The listing builds one solid part. Answer for the finished solid, in the listing's coordinates (mm). Face numbers are marked on the shaded views. A direction names the side the tool comes from. Coordinates: 2 decimals unless noted, no trailing zeros. Loops run counter-clockwise (first coordinate to the right, second up) from the corner with the lowest first, then second, coordinate; pieces in that order, holes last. Notation, with made-up numbers: M -29,-10.75 L -12,-10.75 A18 cw -12,0.25 Z; hole C -17.5,55.5 d5. An arc over 180 degrees is marked long. Answer in a Markdown table with one row per item. Add a question column.
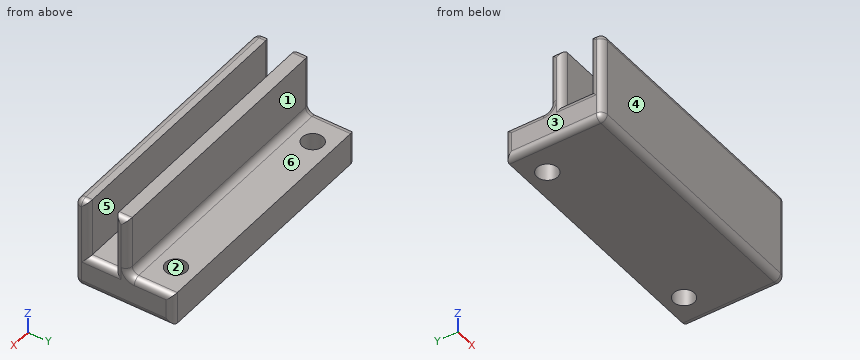
from build123d import *

# Parameters (mm, degrees)
SKETCH2_W           = 40
SKETCH2_H           = 6.9
SKETCH2_R           = 1.6
SKETCH2_H_2         = 2
SKETCH2_H_3         = 4.1
BOSS_EXTRUDE1_DEPTH = 5
SKETCH2_3_W         = 40
SKETCH2_3_H         = 2
BOSS_EXTRUDE2_DEPTH = 14
FILLET1_R           = 1


with BuildPart() as part:
    # Sketch2 → Boss-Extrude1 (new body)
    # profile 1 of 4: a face of its own
    with BuildSketch(Plane.XY):
        with Locations((0, 4.05)):
            Rectangle(SKETCH2_W, SKETCH2_H)
        with Locations((-15, 4.5)):
            Circle(SKETCH2_R, mode=Mode.SUBTRACT)
        with Locations((15, 4.5)):
            Circle(SKETCH2_R, mode=Mode.SUBTRACT)
    # profile 2 of 4: a face of its own
    with BuildSketch(Plane.XY):
        with Locations((0, -0.4)):
            Rectangle(SKETCH2_W, SKETCH2_H_2)
    # profile 3 of 4: a face of its own
    with BuildSketch(Plane.XY):
        with Locations((0, -3.45)):
            Rectangle(SKETCH2_W, SKETCH2_H_3)
    # profile 4 of 4: a face of its own
    with BuildSketch(Plane.XY):
        with Locations((0, -6.5)):
            Rectangle(SKETCH2_W, SKETCH2_H_2)
    extrude(amount=BOSS_EXTRUDE1_DEPTH)

    # Sketch2<3> → Boss-Extrude2 (add)
    with BuildSketch(Plane.XY):
        with Locations((0, -0.4)):
            Rectangle(SKETCH2_3_W, SKETCH2_3_H)
        with Locations((0, -6.5)):
            Rectangle(SKETCH2_3_W, SKETCH2_3_H)
    extrude(amount=BOSS_EXTRUDE2_DEPTH)

    # Fillet1
    fillet1_edges = [part.edges().sort_by_distance(p)[0] for p in [
        (20, 0, 0),
        (0, -7.5, 0),
        (-20, 0, 0),
        (-20, 7.5, 2.5),
        (20, 7.5, 2.5),
        (20, -7.5, 7),
        (-20, -7.5, 7),
        (-20, 4.05, 5),
        (20, 4.05, 5),
        (-20, 0.6, 9.5),
        (-20, -0.4, 14),
        (-20, -1.4, 9.5),
        (20, -1.4, 9.5),
        (20, 0.6, 9.5),
        (0, 0.6, 5),
        (20, -0.4, 14),
        (20, -3.45, 5),
        (-20, -3.45, 5),
        (20, -5.5, 9.5),
        (-20, -5.5, 9.5),
        (-20, -6.5, 14),
        (0, -7.5, 14),
        (20, -6.5, 14),
    ]]
    fillet(fillet1_edges, radius=FILLET1_R - 0.0001)  # a hair under: the kernel refuses the full size


solid = part.part
(1) A cutting plane is placed at A-A (x = 15). Give the vertices of the cut face in (y, z).
(2) A cutting plane is placed at C-C (y = 4.5). Give the vertices of the cut face in (x, z), plus the area to 3 significant figures.
(3) Each of these flat-tipped pins is pushed along its axis until it touches: pin 1 (5 mm diameter, centred on y = 3.5, z = 8.5, fed in from +X); pin 2 (1.2 mm diameter, centred on x = -5.5, y = -4, fed in from +Z); pin 3 (2.5 mm diameter, centred on x = 8.5, z = 9, fed in from +Y). Where does it stop, or does it pass through?
(4) A cutting plane is placed at D-D (x = 7). Give the vertices of the cut face in (y, z).
(5) For the marked faces 4, 5 and 6, determine the directions among +Z, -Z, +X, -X, +Y, -Y from which every point of the face is accessible in a straight line to the end or side of a thin tool.
(6) The mould has two halves that part along X. Classify the marked faces 1, 2 and 3: released by +X, released by -X, zero draft, split by the parting line, or undercut.
(7) Straight lines are drawn through the part: line 1 (Y direction, x = 3.5, z = 13); line 2 (Y direction, x = -15, z = 3.25); line 3 (Z direction, x = 13.5, y = 6). For each, find the intervals that lie inside material, in ascending order.
Solved:
| question | item | result |
|---|---|---|
| 1 | outline | M -7.5,1 A1 ccw -6.5,0 L 2.9,0 L 2.9,5 L 1.6,5 A1 cw 0.6,6 L 0.6,14 L -1.4,14 L -1.4,5 L -5.5,5 L -5.5,14 L -6.5,14 A1 ccw -7.5,13 Z; M 6.1,0 L 7.5,0 L 7.5,5 L 6.1,5 Z |
| 2 | outline | M -20,1 A1 ccw -19,0 L -16.6,0 L -16.6,5 L -19,5 A1 ccw -20,4 Z; M -13.4,0 L 13.4,0 L 13.4,5 L -13.4,5 Z; M 16.6,0 L 19,0 A1 ccw 20,1 L 20,4 A1 ccw 19,5 L 16.6,5 Z |
| 2 | area | 167 mm² |
| 3 | pin 1 | passes through |
| 3 | pin 2 | stops at z = 5 |
| 3 | pin 3 | stops at y = 0.6 |
| 4 | outline | M -7.5,1 A1 ccw -6.5,0 L 7.5,0 L 7.5,5 L 1.6,5 A1 cw 0.6,6 L 0.6,14 L -1.4,14 L -1.4,5 L -5.5,5 L -5.5,14 L -6.5,14 A1 ccw -7.5,13 Z |
| 5 | face 4 | +Z, -Z, +X, -X, -Y |
| 5 | face 5 | +Z, +X, -X |
| 5 | face 6 | +Z, +X, -X, +Y |
| 6 | face 1 | zero draft |
| 6 | face 2 | undercut |
| 6 | face 3 | released by -X |
| 7 | line 1 | y = -7.5 to -5.5, -1.4 to 0.6 |
| 7 | line 2 | y = -7.5 to 2.9, 6.1 to 7.5 |
| 7 | line 3 | z = 0 to 5 |
